Read the model definition and answer for the solid it produces. Units are mm, in the model's axes. A direction names the side the tool comes from. Give positions to 0.01 mm unless a question says otherwise; leave off trailing zeros. Loops run counter-clockwise (first coordinate to the right, second up) from the corner with the lowest first, then second, coordinate; pieces in that order, holes last. Notation, with made-up numbers: (21, -37.75) - (60, -37.75) arc R33 cw to (60, 0.25) - close; hole circle Ø4 at (66.5, 49). An arc over 180 degrees is marked (long way). Write each question's results on one line, items separated by ' | '. Start each with the question number.
Q1. The part is cut by section C-C, the plane z = 8. Write down the section's boundary in (x, y).
Q2. The part is cut by section A-A, the plane y = 4. Write down the section's boundary in (x, z), plus the area to 3 significant figures.
Q3. The part is cut by section B-B, the plane x = 253.5. Write down the section's boundary in (y, z), plus the area to 3 significant figures.
Q4. Determine the mould class of faces 1 (the flat face through (235, 24, 35)), 2 (the flat face through (85, 15, 17)), 3 (the flat face through (179.5, 15, -2)), 4 (the flat face through (234, 13, 40)) for opening direction X: +X half, -X half, draft (parallel to the pull), parting line (faces both ways), or undercut.
Q5. Find the intervals of material crossed by line 1 (Z direction, x = 113.5, y = 30.5); line 2 (Y direction, x = 230, z = 32); line 3 (X direction, y = 13, z = 5), in increasing order. Write a range as from..to.
Q6. Given pin 1 (1.5 mm diameter, centred on y = 13, z = -2.5, fed in from +X); pin 2 (3 mm diameter, centred on y = 36, z = 24, fed in from -X); pin 3 (4 mm diameter, centred on x = 287, z = 30, fed in from +Y); pin 4 (5.5 mm diameter, centred on y = 11.5, z = 37.5, fed in from +X), each flat-ended and moving along its own axis, determine where each tip first touches the part or whether it passes through.
Q7. For faces 5 (the flat face through (184, -5, 17)), 6 (the flat face through (235, 25, 0)), 7 (the flat face through (179.5, 15, 38)), determine the directions among +Z, -Z, +X, -X, +Y, -Y from which every point of the face is accessible in a straight line to the end or side of a thin tool.
Q8. The part is cut by section D-D, the plane y = 15. Write down the section's boundary in (x, z), plus the area to 3 significant figures.
Autodesk Inventor part; units mm, degrees
ref_plane "YZ Plane" through (0, 0, 0) normal (1, 0, 0) x (0, 1, 0)
ref_plane "XZ Plane" through (0, 0, 0) normal (0, 1, 0) x (-1, 0, 0)
ref_plane "XY Plane" through (0, 0, 0) normal (0, 0, 1) x (1, 0, 0)
sketch "Sketch1" plane through (0, 0, 0) normal (0, 0, 1) x (1, 0, 0)
  line L0 (90, 0) -> (280, 0)
  arc A0 (280, 0) -> (376.4181, 35.0933) centre (280, 150) ccw
  line L1 (280, 0) -> (376.4181, 35.0933) construction
  line L2 (0, 0) -> (0, 82.2351) construction
  dimension "d0" = 150
  dimension "d4" = 20
  dimension "d6" = 280
  dimension "d19" = 173.0413
  dimension "d64" = 90
ref_plane "Work Plane1" through (0, 0, 0) normal (1, 0, 0) x (0, 1, 0)
sketch "Sketch2" plane through (0, 0, 0) normal (1, 0, 0) x (0, 1, 0)
  line L0 (0, 0) -> (35, 0)
  line L1 (35, 35) -> (0, 35)
  line L2 (0, 35) -> (0, 0)
  line L3 (35, -5) -> (-5, -5)
  line L4 (-5, -5) -> (-5, 40)
  line L5 (-5, 40) -> (35, 40)
  line L6 (35, -5) -> (35, 0)
  line L7 (35, 35) -> (35, 40)
  dimension "d7" = 35
  dimension "d11" = 35
  dimension "d12" = 90
  dimension "d13" = 35
  dimension "d14" = 40
  dimension "d15" = 45
  dimension "d16" = 35
ref_plane "Work Plane4" through (0, -5, 40) normal (0, 0, 1) x (1, 0, 0)
sketch "Sketch3" plane through (0, -5, 40) normal (0, 0, 1) x (1, 0, 0)
  line L0 (179.5, 0) -> (179.5, 40)
  line L1 (179.5, 40) -> (224.5, 40)
  line L2 (224.5, 40) -> (224.5, 0)
  line L3 (224.5, 0) -> (179.5, 0)
  line L4 (179.5, 5) -> (224.5, 5)
  line L5 (179.5, 35) -> (224.5, 35)
  point P0 (0, 5)
  point P1 (0, 0)
  dimension "d20" = 45
  dimension "d21" = 179.5
  dimension "d65" = 40
  dimension "d66" = 30
  dimension "d67" = 5
  dimension "d68" = 30
ref_plane "Work Plane6" through (0, 0, 35) normal (0, 1, 0) x (1, 0, 0)
sketch "Sketch4" plane through (0, 0, 35) normal (0, 1, 0) x (1, 0, 0)
  point P0 (0, 35)
ref_plane "Work Plane2" through (224.5, 0, 17.5) normal (0, 0, 1) x (1, 0, 0)
sketch "Sketch5" plane through (224.5, 0, 17.5) normal (0, 0, 1) x (1, 0, 0)
  arc A0 (-77.6803, 0) -> (-64.6037, 0) centre (-71.142, 13.5) ccw
  line L0 (-224.5, 0) -> (-35.51, 0)
  line L1 (-224.5, -5) -> (-224.5, 30)
  line L2 (-77.6803, 0) -> (-64.6037, 0)
  line L3 (-71.142, -1.5) -> (-71.142, 0)
  dimension "d44" = 30
  dimension "d45" = 13.5
  dimension "d46" = 153.358
ref_plane "Work Plane7" through (0, 0, 35) normal (0, 1, 0) x (1, 0, 0)
ref_plane "Work Plane5" through (5, 35, 40) normal (0, 1, 0) x (1, 0, 0)
ref_plane "Work Plane3" through (90, 0, 0) normal (1, 0, 0) x (0, 1, 0)
sketch "Sketch8" plane through (90, 0, 0) normal (1, 0, 0) x (0, 1, 0)
  line L0 (31.2631, -5) -> (-5, -5)
  line L1 (35, -5) -> (-5, -5)
  line L2 (-5, -5) -> (-5, 40)
  line L3 (-5, 40) -> (35, 40)
  line L4 (35, 40) -> (35, 35)
  line L5 (35, 35) -> (0, 35)
  line L6 (0, 35) -> (0, 0)
  line L7 (0, 0) -> (35, 0)
  line L8 (35, 0) -> (35, -5)
  dimension "d59" = 45
  dimension "d60" = 40
sweep "Sweep3" add profiles "Sketch8" path "Sketch1"
extrude "Extrusion5" cut sketch "Sketch3" against normal through all contours L0 L5 L2 L4
revolve "Revolution2" cut sketch "Sketch5" angle 360 about axis through (153.358, -1.5, 17.5) along (0, 1, 0) picked at (-67.4817, -0.2757) contours L3 L0 A0
sketch "Sketch9" plane through (90, -5, -5) normal (-1, 0, 0) x (0, 0, 1)
  line L0 (0, 40) -> (0, 0)
  line L1 (0, 0) -> (45, 0)
  line L2 (45, 0) -> (45, 40)
  line L3 (45, 40) -> (40, 40)
  line L4 (40, 40) -> (0, 40)
  point P0 (5, 5)
  dimension "d74" = 45
  dimension "d75" = 5
extrude "Extrusion6" add sketch "Sketch9" along normal blind 5
properties part number "Shooting Ramp"
Check sheet entries:
1) outline: (85, -5) - (280, -5) arc R155 ccw to (379.63, 31.26) - (376.42, 35.09) arc R150 cw to (280, 0) - (90, 0) - (90, 35) - (85, 35) - close
2) outline: (85, -5) - (179.5, -5) - (179.5, 0) - (90, 0) - (90, 35) - (179.5, 35) - (179.5, 40) - (85, 40) - close; (224.5, -5) - (332.05, -5) - (332.05, 40) - (224.5, 40) - (224.5, 35) - (314.41, 35) - (314.41, 0) - (224.5, 0) - close | area: 2,810 mm^2
3) outline: (-5, -5) - (35, -5) - (35, 0) - (0, 0) - (0, 35) - (35, 35) - (35, 40) - (-5, 40) - close | area: 575 mm^2
4) face 1: undercut | face 2: -X half | face 3: undercut | face 4: draft
5) line 1: z = -5..0, 35..40 | line 2: y = -5..0 | line 3: x = 85..90, 341.08..352.5
6) pin 1: stops at x = 353.9 | pin 2: stops at x = 85 | pin 3: stops at y = 0.27 | pin 4: stops at x = 354.81
7) face 5: +Z, -Z, +X, -X, -Y | face 6: +Y | face 7: +Z, -Z
8) outline: (85, -5) - (179.5, -5) - (179.5, 0) - (90, 0) - (90, 35) - (179.5, 35) - (179.5, 40) - (85, 40) - close; (224.5, -5) - (356.16, -5) - (356.16, 40) - (224.5, 40) - (224.5, 35) - (345.38, 35) - (345.38, 0) - (224.5, 0) - close | area: 2,810 mm^2
